Check sheet for the modelled part. Datum: model origin and axes. Units: mm. Give positions to 0.01 mm unless a question says otherwise; leave off trailing zeros. Write each loop counter-clockwise with the first axis right and the second up, starting at its lowest first coordinate (ties: lowest second). Pieces come first, ordered by that corner, then holes.
from build123d import *

# Parameters (mm, degrees)
SKETCH1_W           = 130
SKETCH1_H           = 76.5
SKETCH1_R           = 12
SKETCH1_R_2         = 1.8
SKETCH1_W_2         = 56.5
SKETCH1_H_2         = 56.5
SKETCH1_W_3         = 28
SKETCH1_H_3         = 28
SKETCH1_W_4         = 2.65
SKETCH1_H_4         = 30
BOSS_EXTRUDE1_DEPTH = 3.175
FILLET1_R           = 5


with BuildPart() as part:
    # Sketch1 → Boss-Extrude1 (new body)
    with BuildSketch(Plane(origin=(0, 0, 0), x_dir=(1, 0, 0), z_dir=(0, 1, 0))):
        with Locations((65, 38.25)):
            Rectangle(SKETCH1_W, SKETCH1_H)
        with Locations(Location((100, 17, 0), (0, 0, 270))):
            Circle(SKETCH1_R, mode=Mode.SUBTRACT)
        with Locations(Location((119, 17, 0), (0, 0, 270))):
            Circle(SKETCH1_R_2, mode=Mode.SUBTRACT)
        with Locations(Location((81, 17, 0), (0, 0, 90))):
            Circle(SKETCH1_R_2, mode=Mode.SUBTRACT)
        with Locations((38.25, 38.25)):
            Rectangle(SKETCH1_W_2, SKETCH1_H_2, mode=Mode.SUBTRACT)
        with Locations((98.35, 55)):
            Rectangle(SKETCH1_W_3, SKETCH1_H_3, mode=Mode.SUBTRACT)
        with Locations((123.675, 51.5)):
            Rectangle(SKETCH1_W_4, SKETCH1_H_4, mode=Mode.SUBTRACT)
    extrude(amount=BOSS_EXTRUDE1_DEPTH)

    # Fillet1
    fillet1_edges = [part.edges().sort_by_distance(p)[0] for p in [
        (0, 1.5875, -76.5),
        (130, 1.5875, -76.5),
        (130, 1.5875, 0),
        (0, 1.5875, 0),
    ]]
    fillet(fillet1_edges, radius=FILLET1_R)


solid = part.part
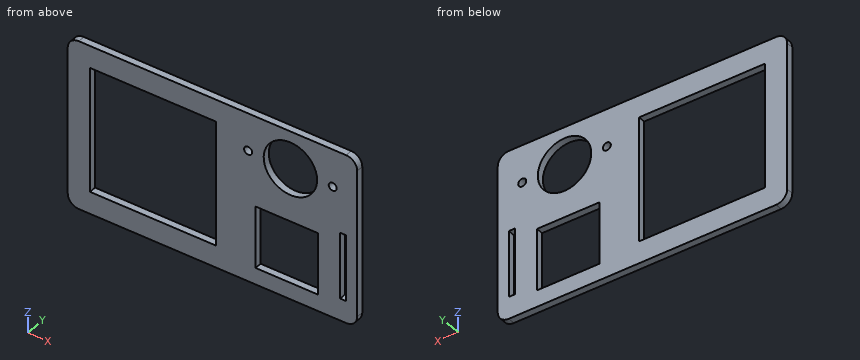
1) Sectioned sample at D-D on z = -17. Record the boundary of the cut face in (x, y) (3 decimals), then the cut area to 3 significant figures.
2) Sectioned sample at A-A on x = 20.5. Record the boundary of the cut face in (y, z) (3 decimals).
3) Scan lines: L1, parallel to X at y = 2.45, z = -38.5; L2, parallel to X at y = 2.25, z = -17; L3, parallel to X at y = 0.75, z = -45.5. Record each from-to range of solid material in increasing order.
4) Sectioned sample at C-C on z = -60.5. Record the boundary of the cut face in (x, y) (3 decimals), then the cut area to 3 significant figures.
5) Sectioned sample at B-B on y = 1.1. Record the boundary of the cut face in (x, z), then the cut area to 3 significant figures.
Answers below:
1. outline: (0, 0) - (10, 0) - (10, 3.175) - (0, 3.175) - close; (66.5, 0) - (79.2, 0) - (79.2, 3.175) - (66.5, 3.175) - close; (82.8, 0) - (88, 0) - (88, 3.175) - (82.8, 3.175) - close; (112, 0) - (117.2, 0) - (117.2, 3.175) - (112, 3.175) - close; (120.8, 0) - (130, 0) - (130, 3.175) - (120.8, 3.175) - close
1. area: 134 mm2
2. outline: (0, -76.5) - (3.175, -76.5) - (3.175, -66.5) - (0, -66.5) - close; (0, -10) - (3.175, -10) - (3.175, 0) - (0, 0) - close
3. L1: x = 0 to 10, 66.5 to 122.35, 125 to 130
3. L2: x = 0 to 10, 66.5 to 79.2, 82.8 to 88, 112 to 117.2, 120.8 to 130
3. L3: x = 0 to 10, 66.5 to 84.35, 112.35 to 122.35, 125 to 130
4. outline: (0, 0) - (10, 0) - (10, 3.175) - (0, 3.175) - close; (66.5, 0) - (84.35, 0) - (84.35, 3.175) - (66.5, 3.175) - close; (112.35, 0) - (122.35, 0) - (122.35, 3.175) - (112.35, 3.175) - close; (125, 0) - (130, 0) - (130, 3.175) - (125, 3.175) - close
4. area: 136 mm2
5. outline: (0, -71.5) arc R5 ccw to (5, -76.5) - (125, -76.5) arc R5 ccw to (130, -71.5) - (130, -5) arc R5 ccw to (125, 0) - (5, 0) arc R5 ccw to (0, -5) - close; hole (10, -66.5) - (66.5, -66.5) - (66.5, -10) - (10, -10) - close; hole circle Ø3.6 at (81, -17); hole (84.35, -69) - (112.35, -69) - (112.35, -41) - (84.35, -41) - close; hole circle Ø24 at (100, -17); hole circle Ø3.6 at (119, -17); hole (122.35, -66.5) - (125, -66.5) - (125, -36.5) - (122.35, -36.5) - close
5. area: 5,400 mm2
